from build123d import *

# Parameters (mm, degrees)
BOSS_EXTRUDE1_DEPTH = 6.35
SKETCH2_R           = 1.0414
CUT_EXTRUDE1_DEPTH  = 31.496215156
SKETCH3_R           = 1.0414
CUT_EXTRUDE2_DEPTH  = 30.82342263


with BuildPart() as part:
    # Sketch1 → Boss-Extrude1 (new body)
    with BuildSketch(Plane(origin=(0, 0, 0), x_dir=(1, 0, 0), z_dir=(0, 1, 0))):
        Polygon((-16.681663134, -25.179419289), (-16.681663134, -17.559419289), (-23.400364211, -7.62), (-23.400364211, 0), (-23.400364211, 3.175), (-25.940364211, 3.175), (-25.940364211, 0), (-25.940364211, -7.62), (-19.221663134, -17.559419289), (-19.221663134, -25.179419289), (-19.221663134, -28.354419289), (-16.681663134, -28.354419289), align=None)
    extrude(amount=BOSS_EXTRUDE1_DEPTH)

    # Sketch2 → Cut-Extrude1 (cut, through all)
    with BuildSketch(Plane.ZY.offset(25.940364211)):
        with BuildLine():
            ThreePointArc((-3.175, 3.175), (-2.24506403, 5.42006403), (0, 6.35))
            Line((0, 6.35), (-3.175, 6.35))
            Line((-3.175, 6.35), (-3.175, 3.175))
        make_face()
        with BuildLine():
            ThreePointArc((0, 0), (-2.24506403, 0.92993597), (-3.175, 3.175))
            Line((-3.175, 3.175), (-3.175, 0))
            Line((-3.175, 0), (0, 0))
        make_face()
        with Locations((0, 3.175)):
            Circle(SKETCH2_R)
    extrude(amount=-CUT_EXTRUDE1_DEPTH, mode=Mode.SUBTRACT)

    # Sketch3 → Cut-Extrude2 (cut, through all)
    with BuildSketch(Plane.ZY.offset(19.221663134)):
        with BuildLine():
            Line((28.354419289, 6.35), (25.179419289, 6.35))
            ThreePointArc((25.179419289, 6.35), (27.424483319, 5.42006403), (28.354419289, 3.175))
            Line((28.354419289, 3.175), (28.354419289, 6.35))
        make_face()
        with BuildLine():
            Line((28.354419289, 0), (28.354419289, 3.175))
            ThreePointArc((28.354419289, 3.175), (27.424483319, 0.92993597), (25.179419289, 0))
            Line((25.179419289, 0), (28.354419289, 0))
        make_face()
        with Locations((25.179419289, 3.175)):
            Circle(SKETCH3_R)
    extrude(amount=-CUT_EXTRUDE2_DEPTH, mode=Mode.SUBTRACT)


solid = part.part
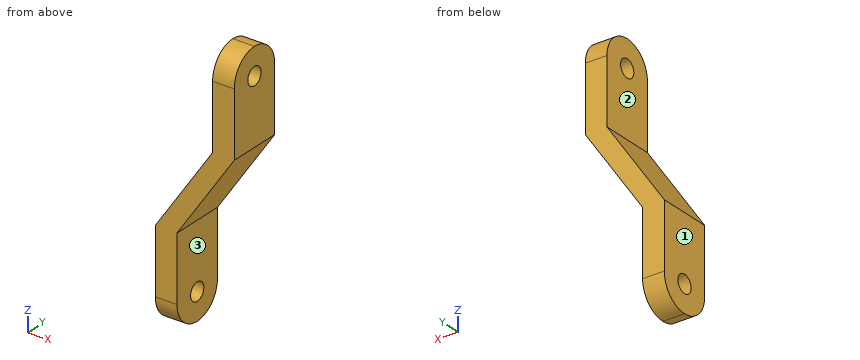
The listing builds one solid part. Answer for the finished solid, in the listing's coordinates (mm). Face numbers are marked on the shaded views. A direction names the side the tool comes from. Round coordinates to 2 decimals unless told otherwise and drop trailing zeros. Order: outer loops, then holes, each group sorted by start corner. A loop starts at its lowest first (then second) coordinate and runs counter-clockwise, first axis right, second up. Notation, with made-up numbers: (11, -10.5) - (17, -10.5) arc R24 cw to (17, 25.5) - close; hole circle Ø11 at (22, -22.5). An arc over 180 degrees is marked (long way). Write item = value, one per line. Start each with the question number.
1) For the marked faces 1, 2 and 3, determine the directions among +Z, -Z, +X, -X, +Y, -Y from which every point of the face is accessible in a straight line to the end or side of a thin tool.
2) Section B-B, the plane x = -23.75 is taken. Write down the section's boundary in (y, z) (3 decimals), plus the area to 3 significant figures.
3) Straight lines are drawn through the part: L1, parallel to Y at x = -24.45, z = 0; L2, parallel to X at y = 1.5, z = 25.5; L3, parallel to X at y = 3.75, z = 1. For each, find the intervals that lie inside material, in ascending order.
4) Given pin 1 (2 mm diameter, centred on y = 1, z = 1.5, fed in from +X), flat-ended and moving along its own axis, determine where the tip first touches the part or whether it passes through.
5) Section A-A, the plane y = 2.5 is taken. Write down the section's boundary in (x, z).
6) Section D-D, the plane z = 1.5 is taken. Write down the section's boundary in (x, y).
7) Section C-C, the plane y = 5.25 is taken. Write down the section's boundary in (x, z).
Results list:
q1.face_1 = +Z, -Z, -X, +Y, -Y
q1.face_2 = +Z, -X, +Y, -Y
q1.face_3 = -Z, +X, +Y, -Y
q2.outline = (0, 0) arc R3.175 ccw to (6.35, 0) - (6.35, 10.86) - (0, 10.86) - close; hole circle Ø2.083 at (3.175, 0)
q2.area = 81.4 mm^2
q3.L1 = 0 to 2.13, 4.22 to 6.35
q3.L2 = -19.22 to -16.68
q3.L3 = -25.94 to -23.4
q4.pin_1 = -23.4
q5.outline = (-25.94, -3.1) - (-23.4, -3.1) - (-23.4, -0.79) - (-25.94, -0.79) - close; (-25.94, 0.79) - (-23.4, 0.79) - (-23.4, 7.62) - (-16.68, 17.56) - (-16.68, 24.39) - (-19.22, 24.39) - (-19.22, 17.56) - (-25.94, 7.62) - close; (-19.22, 25.97) - (-16.68, 25.97) - (-16.68, 28.28) - (-19.22, 28.28) - close
q6.outline = (-25.94, 0) - (-23.4, 0) - (-23.4, 6.35) - (-25.94, 6.35) - close
q7.outline = (-25.94, -2.4) - (-23.4, -2.4) - (-23.4, 7.62) - (-16.68, 17.56) - (-16.68, 27.58) - (-19.22, 27.58) - (-19.22, 17.56) - (-25.94, 7.62) - close
